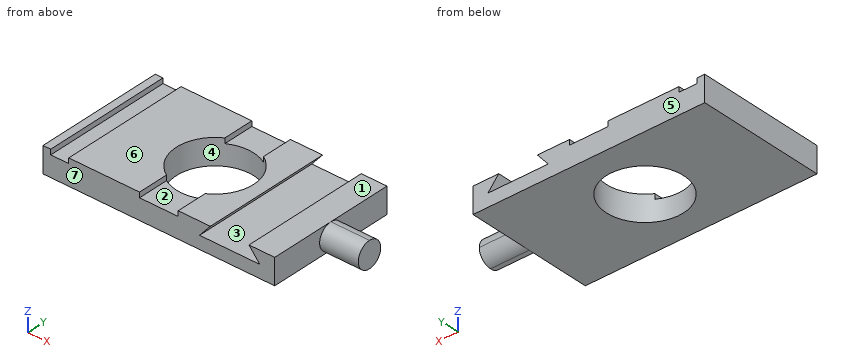
```python
from build123d import *

# Parameters (mm, degrees)
F0_W     = 89.999996
F0_H     = 50
F0_R     = 15
F1_DEPTH = 10
F2_W     = 7
F2_H     = 50
F3_DEPTH = 2
F5_DEPTH = 50.001
F7_DEPTH = 15


with BuildPart() as f1:
    # F0 (on Top) → F1 (new body)
    with BuildSketch(Plane.XY):
        Rectangle(F0_W, F0_H)
        Circle(F0_R, mode=Mode.SUBTRACT)
    extrude(amount=F1_DEPTH)

    # F2 (on face) → F3 (cut)
    with BuildSketch(Plane.XY.offset(10)):
        with Locations((-38.499998, 0)):
            Rectangle(F2_W, F2_H)
        with BuildLine():
            Line((-7.5, -12.990381), (-7.5, -25))
            Line((-7.5, -25), (7.5, -25))
            Line((7.5, -25), (7.5, -12.990381))
            ThreePointArc((7.5, -12.990381), (0, -15), (-7.5, -12.990381))
        make_face()
        with BuildLine():
            Line((7.5, 25), (-7.5, 25))
            Line((-7.5, 25), (-7.5, 12.990381))
            ThreePointArc((-7.5, 12.990381), (0, 15), (7.5, 12.990381))
            Line((7.5, 12.990381), (7.5, 25))
        make_face()
    extrude(amount=-F3_DEPTH, mode=Mode.SUBTRACT)

    # F4 (on face) → F5 (cut, through all)
    with BuildSketch(Plane.XZ.offset(25)):
        Polygon((35, 10), (20, 10), (15.804502, 5), (39.195498, 5), align=None)
    extrude(amount=-F5_DEPTH, mode=Mode.SUBTRACT)

    # F6 (on face) → F7 (join)
    with BuildSketch(Plane.YZ.offset(44.999998)):
        with BuildLine():
            ThreePointArc((0, 0), (3.535534, 1.464466), (5, 5))
            ThreePointArc((5, 5), (3.535534, 8.535534), (0, 10))
            ThreePointArc((0, 10), (-5, 5), (0, 0))
        make_face()
    extrude(amount=F7_DEPTH)


solid = f1.part
```
Can you work these out from the model? Positions are in its coordinate system, mm. Face numbers are marked on the shaded views. A direction names the side the tool comes from. Coordinates: 2 decimals unless noted, no trailing zeros. Loops run counter-clockwise (first coordinate to the right, second up) from the corner with the lowest first, then second, coordinate; pieces in that order, holes last. Notation, with made-up numbers: (67.5, -31.75) -> (84.5, -31.75) arc R22 ccw to (84.5, -22.75) -> close; hole circle Ø7 at (81.5, 4). An arc over 180 degrees is marked (long way). Answer as a JSON object with one key per item and string values.
1) For P1, Ø5, axis at y = 17.5, z = 3, coming from the +X side; P2, Ø3.5, axis at x = -38.5, y = -12, coming from the +Z side; P3, Ø1, axis at x = 27.5, y = 16, coming from the +Z side; P4, Ø4, axis at x = -10, y = 5, coming from the +Z side, each with a flat end and sliding along its axis, tell me the tip position at first contact or that it passes through.
Results:
{"P1": "stops at x = 45", "P2": "stops at z = 8", "P3": "stops at z = 5", "P4": "passes through"}
2) Thinking about a two-plate mould opening in Y: for the marked faces 4, 5, 6 and 7, which applies, pulls with the +Y half, pulls with the -Y half, needs draft (parallel to the pull), parting line crosses it, or undercut?
Results:
{"face 4": "undercut", "face 5": "pulls with the +Y half", "face 6": "needs draft", "face 7": "pulls with the -Y half"}
3) Imagine slicing it at B-B (x = 0). Please give me the cut outline in (y, z).
Results:
{"outline": "(-25, 0) -> (-15, 0) -> (-15, 8) -> (-25, 8) -> close; (15, 0) -> (25, 0) -> (25, 8) -> (15, 8) -> close"}
4) Imagine slicing it at A-A (z = 6). Please give me the cut outline in (x, y).
Results:
{"outline": "(-45, -25) -> (16.64, -25) -> (16.64, 25) -> (-45, 25) -> close; (38.36, -25) -> (45, -25) -> (45, -4.9) -> (60, -4.9) -> (60, 4.9) -> (45, 4.9) -> (45, 25) -> (38.36, 25) -> close; hole circle Ø30 at (0, 0)"}
5) Imagine slicing it at D-D (y = 16). Please give me the cut outline in (x, z), then the cut area to 3 significant figures.
Results:
{"outline": "(-45, 0) -> (45, 0) -> (45, 10) -> (35, 10) -> (39.2, 5) -> (15.8, 5) -> (20, 10) -> (7.5, 10) -> (7.5, 8) -> (-7.5, 8) -> (-7.5, 10) -> (-35, 10) -> (-35, 8) -> (-42, 8) -> (-42, 10) -> (-45, 10) -> close", "area": "760 mm^2"}
6) Imagine slicing it at C-C (y = -4). Please give me the cut outline in (x, z), then the cut area to 3 significant figures.
Results:
{"outline": "(-45, 0) -> (-14.46, 0) -> (-14.46, 10) -> (-35, 10) -> (-35, 8) -> (-42, 8) -> (-42, 10) -> (-45, 10) -> close; (14.46, 0) -> (45, 0) -> (45, 2) -> (60, 2) -> (60, 8) -> (45, 8) -> (45, 10) -> (35, 10) -> (39.2, 5) -> (15.8, 5) -> (20, 10) -> (14.46, 10) -> close", "area": "591 mm^2"}
7) For the marked faces 1, 2 and 3, which set-ups out of +Z, -Z, +X, -X, +Y, -Y let a thin tool reach every point of the face, with its end or its side?
Results:
{"face 1": "+Z, +X, -X, +Y, -Y", "face 2": "+Z, +Y, -Y", "face 3": "+Y, -Y"}
8) If I drill on line 1 (Y direction, x = 0, z = 6); line 2 (X direction, y = -13, z = 2.5); line 3 (X direction, y = 15.5, z = 8.25), over which ranges is the centre line in solid material (lowest first)?
Results:
{"line 1": "y = -25 to -15, 15 to 25", "line 2": "x = -45 to -7.48, 7.48 to 45", "line 3": "x = -45 to -42, -35 to -7.5, 7.5 to 18.53, 36.47 to 45"}
